```python
from build123d import *

# Parameters (mm, degrees)
BOSS_EXTRUDE1_DEPTH = 60
FILLET1_R           = 5
CHAMFER1_SIZE       = 2


with BuildPart() as part:
    # Sketch1 → Boss-Extrude1 (new body)
    with BuildSketch(Plane.XY):
        Polygon((40, 12.5), (43, 12.5), (43, -12.5), (-43, -12.5), (-43, 12.5), (-40, 12.5), (-40, 2.5), (40, 2.5), align=None)
    extrude(amount=BOSS_EXTRUDE1_DEPTH)

    # Fillet1
    fillet1_edges = [part.edges().sort_by_distance(p)[0] for p in [
        (-40, 2.5, 30),
        (40, 2.5, 30),
    ]]
    fillet(fillet1_edges, radius=FILLET1_R)

    # Chamfer1
    chamfer1_edges = [part.edges().sort_by_distance(p)[0] for p in [
        (-43, 12.5, 30),
        (43, 12.5, 30),
    ]]
    chamfer(chamfer1_edges, length=CHAMFER1_SIZE)


solid = part.part
```
Input: part model. Units: mm. Frame: model coordinates. A direction names the side the tool comes from. Round coordinates to 2 decimals unless told otherwise and drop trailing zeros. Loops run counter-clockwise (first coordinate to the right, second up) from the corner with the lowest first, then second, coordinate; pieces in that order, holes last. Notation, with made-up numbers: (4, -28) -> (55, -28) arc R22 cw to (55, 0) -> close; hole circle Ø10 at (23, 32). An arc over 180 degrees is marked (long way). Use one line per item in the form item = value. Start each with the question number.
Item 1: Mould query, pull axis X, two halves, no side actions, for faces 1 (the face through (1, -5, 60)), 2 (the face through (-38.57, 4, 30.42)), 3 (the face through (-43, -1, 30)). Classes: pulls with the +X half, pulls with the -X half, needs draft (parallel to the pull), parting line crosses it, or undercut.
Item 2: Section query B-B on x = -30. Return the cut outline in (y, z), then the cut area to 3 significant figures.
Item 3: Set-up query: faces 4 (the face through (1, -5, 0)), 5 (the face through (-40, 10, 30)). Return all of +Z, -Z, +X, -X, +Y, -Y with unobstructed straight access to the full face (end or side cutting, diameter ignored); none if empty.
Item 4: Section query A-A on z = 4. Return the cut outline in (x, y), then the cut area to 3 significant figures.
Item 5: Material intervals for L1, parallel to X at y = 7.75, z = 39; L2, parallel to Y at x = -34.5, z = 44; L3, parallel to X at y = 4.5, z = 46, sorted ascending. Write a range as from..to.
Ans:
q1.face_1 = needs draft
q1.face_2 = undercut
q1.face_3 = pulls with the -X half
q2.outline = (-12.5, 0) -> (2.5, 0) -> (2.5, 60) -> (-12.5, 60) -> close
q2.area = 900 mm^2
q3.face_4 = -Z, +X, -X, +Y, -Y
q3.face_5 = +Z, -Z, +Y
q4.outline = (-43, -12.5) -> (43, -12.5) -> (43, 10.5) -> (41, 12.5) -> (40, 12.5) -> (40, 7.5) arc R5 cw to (35, 2.5) -> (-35, 2.5) arc R5 cw to (-40, 7.5) -> (-40, 12.5) -> (-41, 12.5) -> (-43, 10.5) -> close
q4.area = 1,360 mm^2
q5.L1 = -43..-40, 40..43
q5.L2 = -12.5..2.5
q5.L3 = -43..-39, 39..43
